Input: part model. Units: mm. Frame: model coordinates. A direction names the side the tool comes from. Give positions to 0.01 mm unless a question says otherwise; leave off trailing zeros. Loops run counter-clockwise (first coordinate to the right, second up) from the corner with the lowest first, then second, coordinate; pieces in that order, holes last. Notation, with made-up numbers: M 83.5,-2.75 L 137.5,-2.75 A25 ccw 137.5,32.25 Z; hole C 63,-36.5 d10. An arc over 180 degrees is marked long. One line per item, written item: value. Start each with the question number.
(1) Access query for faces 5 (the flat face through (15.86, 4.96, -4.13)), 6 (the cylindrical face through (16.22, 9.4, -4.96)), 7 (the cylindrical face through (-3.817, 0.601, 16.524)). Directions: +Z, -Z, +X, -X, +Y, -Y. A direction counts if a zero-diameter tool reaches every point of the face in a straight line with its end or side. Return the directions, or none.
(2) Pin query (flat end, axial travel): P1, Ø4, axis at x = -20.5, y = 2, coming from the -Z side; P2, Ø4, axis at x = 20, y = 6, coming from the +Z side; P3, Ø2, axis at x = -39, y = 2.5, coming from the -Z side. Return the tip coordinate at first contact, or that it passes through.
(3) Ray query, line 1 along Z through (x, y) = (-3, 5.5); line 2 along Z through (x, y) = (-22, 8.75); line 3 along X through (y, z) = (3, 0.5). Return the intervals inside material, ascending. Write a range as from..to.
(4) Section A-A on y = 4. Output: boundary loops of the cut face in (x, z) (3 decimals), plus the area to 3 significant figures.
(5) Pull-direction query (Z, two-part tool) for faces 1 (the cylindrical face through (-48.84, 5.04, 13.86)), 2 (the cylindrical face through (12.471, 5.042, -49.214)), 3 (the flat face through (-7.039, 4.958, 25.435)), 4 (the flat face through (-4.35, 4.96, 15.8)); classes: released by +Z, released by -Z, zero draft, split by the parting line, or undercut.
```python
from build123d import *

# Parameters (mm, degrees)
EXTRUDE1_DEPTH = 10
FILLET1_R      = 2


with BuildPart() as part:
    # Sketch1 → Extrude1 (new body)
    with BuildSketch(Plane(origin=(0, 0, 0), x_dir=(1, 0, 0), z_dir=(0, 1, 0))):
        Polygon((37.839987617, -36.780043986), (12.932458636, 51.160412548), (-50.772446253, -14.380368562), align=None)
        Polygon((23.498416155, -22.840197215), (8.030982938, 31.770323946), (-31.529399093, -8.930126731), align=None, mode=Mode.SUBTRACT)
    extrude(amount=EXTRUDE1_DEPTH)

    # Fillet1
    fillet1_edges = [part.edges().sort_by_distance(p)[0] for p in [
        (-18.919993808, 10, -18.390021993),
        (-4.015491469, 0, 15.885161973),
        (-31.529399093, 5, 8.930126731),
        (15.764699546, 0, -4.465063366),
        (23.498416155, 5, 22.840197215),
        (-11.749208077, 0, -11.420098607),
        (8.030982938, 5, -31.770323946),
        (-4.015491469, 10, 15.885161973),
        (15.764699546, 10, -4.465063366),
        (-11.749208077, 10, -11.420098607),
        (-18.919993808, 0, -18.390021993),
        (-6.466229318, 10, 25.580206274),
        (25.386223126, 0, -7.190184281),
        (-6.466229318, 0, 25.580206274),
        (-50.772446253, 5, 14.380368562),
        (12.932458636, 5, -51.160412548),
        (37.839987617, 5, 36.780043986),
        (25.386223126, 10, -7.190184281),
    ]]
    fillet(fillet1_edges, radius=FILLET1_R)


solid = part.part
```
Output values:
1. face 5: +Y, -Y
1. face 6: +Y
1. face 7: -Y
2. P1: stops at z = -18.82
2. P2: stops at z = 32.78
2. P3: stops at z = 1.24
3. line 1: z = -34.77..-20.42, 16.14..26.46
3. line 2: z = -15.01..-1.08, 11.49..21.5
3. line 3: x = -37.28..-23.34, 17.17..27.56
4. outline: M -48.358,11.896 L 10.518,-48.676 A2 ccw 13.876,-47.827 L 36.896,33.447 A2 ccw 34.482,35.931 L -47.414,15.229 A2 ccw Z; hole M -29.115,6.446 L 5.617,-29.286 A2 ccw 8.975,-28.437 L 22.554,19.507 A2 ccw 20.14,21.991 L -28.171,9.779 A2 ccw Z
4. area: 2,220 mm²
5. face 1: split by the parting line
5. face 2: released by -Z
5. face 3: released by +Z
5. face 4: undercut
